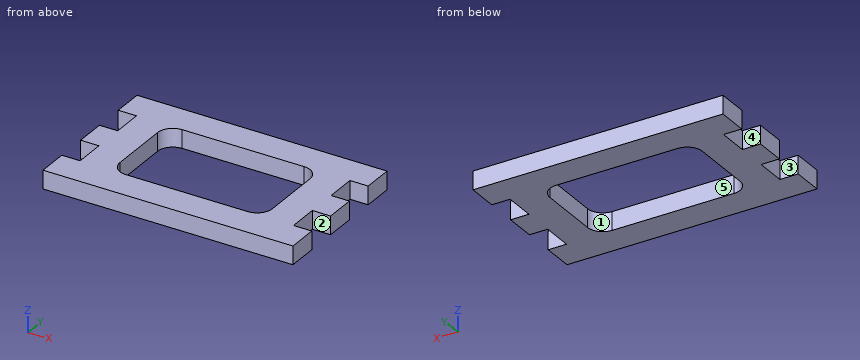
Autodesk Inventor part; units mm, degrees
ref_plane "YZ Plane" through (0, 0, 0) normal (1, 0, 0) x (0, 1, 0)
ref_plane "XZ Plane" through (0, 0, 0) normal (0, 1, 0) x (-1, 0, 0)
ref_plane "XY Plane" through (0, 0, 0) normal (0, 0, 1) x (1, 0, 0)
sketch "Sketch1" plane through (0, 0, 0) normal (0, 0, 1) x (1, 0, 0)
  line L0 (-82, -50) -> (82, -50)
  line L1 (82, -50) -> (82, 50)
  line L2 (82, 50) -> (-82, 50)
  line L3 (-82, 50) -> (-82, -50)
  line L4 (-82, -50) -> (82, 50) construction
  line L5 (82, -50) -> (-82, 50) construction
  point P0 (0, 0)
  dimension "d0" = 164
  dimension "d1" = 100
extrude "Extrusion1" add sketch "Sketch1" along normal mid plane 12
sketch "Sketch2" plane through (0, 0, 6) normal (0, 0, 1) x (1, 0, 0)
  line L0 (-82, 50) -> (-82, -50)
  line L1 (-82, -30) -> (-70, -30)
  line L2 (-70, -30) -> (-70, -10)
  line L3 (-70, -10) -> (-82, -10)
  line L4 (-82, -10) -> (-82, -30)
  line L5 (-82, -50) -> (82, -50)
  line L6 (-82, 10) -> (-70, 10)
  line L7 (-70, 10) -> (-70, 30)
  line L8 (-70, 30) -> (-82, 30)
  line L9 (-82, 30) -> (-82, 10)
  point P0 (0, 0)
  dimension "d4" = 12
  dimension "d5" = 20
  dimension "d6" = 20
  dimension "d7" = 20
  dimension "d8" = 20
extrude "Extrusion2" cut sketch "Sketch2" against normal through all
mirror "Mirror1" about plane through (0, 0, 0) normal (1, 0, 0) of "Extrusion2"
sketch "Sketch3" plane through (0, 0, 6) normal (0, 0, 1) x (1, 0, 0)
  line L0 (-40, -30) -> (40, -30)
  line L1 (50, -20) -> (50, 20)
  line L2 (40, 30) -> (-40, 30)
  line L3 (-50, 20) -> (-50, -20)
  line L4 (-50, -30) -> (50, 30) construction
  line L5 (50, -30) -> (-50, 30) construction
  arc A0 (-40, 30) -> (-50, 20) centre (-40, 20) ccw
  arc A1 (50, 20) -> (40, 30) centre (40, 20) ccw
  arc A2 (40, -30) -> (50, -20) centre (40, -20) ccw
  arc A3 (-50, -20) -> (-40, -30) centre (-40, -20) ccw
  point P0 (0, 0)
  dimension "d11" = 100
  dimension "d12" = 60
  dimension "d13" = 10
  dimension "d14" = 10
extrude "Extrusion3" cut sketch "Sketch3" against normal through all
properties part number "FRONT V2" material "Wood (Cherry)"
Here's how the part is built. I have some questions about the finished solid (model axes, mm). Face numbers are marked on the shaded views. A direction names the side the tool comes from. Coordinates: 2 decimals unless noted, no trailing zeros. Order: outer loops, then holes, each group sorted by start corner. A loop starts at its lowest first (then second) coordinate and runs counter-clockwise, first axis right, second up. Notation, with made-up numbers: M 8.25,89.25 L 53.25,89.25 A19 cw 53.25,106.25 Z; hole C -25.75,32 d5. An arc over 180 degrees is marked long. Answer as a JSON object with one key per item and string values. Group by question number.
(1) Which directions (+Z, -Z, +X, -X, +Y, -Y) give clear straight access to the entire face, cutting with the end or side of a thin tool? Please do the marked faces 1, 2 and 3.
(2) Suppose I cut it at B-B, the plane x = 36. Please give me the cut outline in (y, z), then the cut area to 3 significant figures.
(3) If we mould it in two halves opening along X, with no side actions, what happens to the marked faces 4 and 5? For each: released by +X, released by -X, zero draft, split by the parting line, or undercut.
(4) I need wall thicknesses on probe 1 along Y at (x, z) = (-74, -0.5); probe 2 along X at (y, z) = (4, 3.25); probe 3 along Y at (x, z) = (8.5, -1). Which ranges of each line are inside material? Lowest first, please.
(5) For pin 1 (6 mm diameter, centred on y = 21.5, z = -1.5, fed in from +X); pin 2 (3.5 mm diameter, centred on y = 16.5, z = -1, fed in from -X), each with a flat end and sliding along its axis, tell me the tip position at first contact or that it passes through.
(6) Suppose I cut it at A-A, the plane y = -7.5. Please give me the cut outline in (x, z), then the cut area to 3 significant figures.
(7) Suppose I cut it at C-C, the plane z = -3.75. Please give me the cut outline in (x, y), then the cut area to 3 significant figures.
Values found:
{
 "1": {"face 1": "+Z, -Z", "face 2": "+Z, -Z, +X", "face 3": "+Z, -Z, -X"},
 "2": {"outline": "M -50,-6 L -30,-6 L -30,6 L -50,6 Z; M 30,-6 L 50,-6 L 50,6 L 30,6 Z", "area": "480 mm^2"},
 "3": {"face 4": "zero draft", "face 5": "undercut"},
 "4": {"probe 1": "y = -50 to -30, -10 to 10, 30 to 50", "probe 2": "x = -82 to -50, 50 to 82", "probe 3": "y = -50 to -30, 30 to 50"},
 "5": {"pin 1": "stops at x = 70", "pin 2": "stops at x = -70"},
 "6": {"outline": "M -82,-6 L -50,-6 L -50,6 L -82,6 Z; M 50,-6 L 82,-6 L 82,6 L 50,6 Z", "area": "768 mm^2"},
 "7": {"outline": "M -82,-50 L 82,-50 L 82,-30 L 70,-30 L 70,-10 L 82,-10 L 82,10 L 70,10 L 70,30 L 82,30 L 82,50 L -82,50 L -82,30 L -70,30 L -70,10 L -82,10 L -82,-10 L -70,-10 L -70,-30 L -82,-30 Z; hole M -50,-20 A10 ccw -40,-30 L 40,-30 A10 ccw 50,-20 L 50,20 A10 ccw 40,30 L -40,30 A10 ccw -50,20 Z", "area": "9,530 mm^2"}
}
